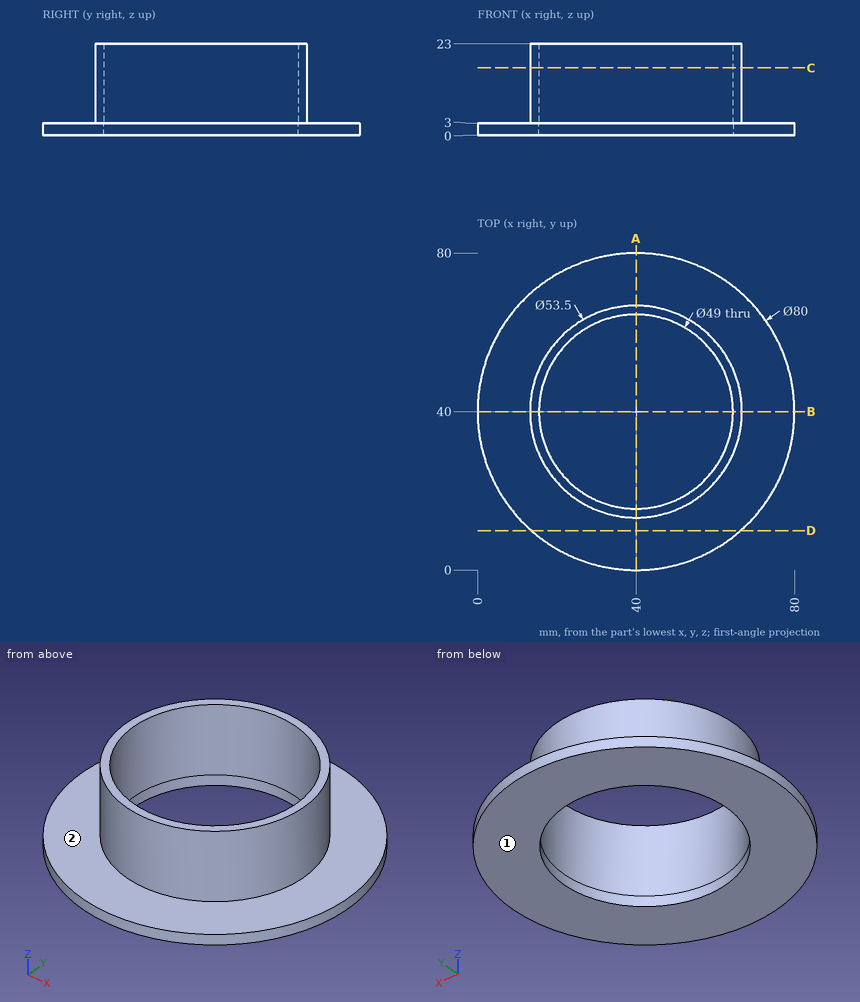
Geometry check sheet. Reference: drawing and pictorial views, mm from the part's lowest x, y, z. A direction names the side the tool comes from. Give positions to 0.01 mm unless a question says otherwise; leave off trailing zeros. Loops run counter-clockwise (first coordinate to the right, second up) from the corner with the lowest first, then second, coordinate; pieces in that order, holes last. Notation, with made-up numbers: (-30, 72.5) - (22, 72.5) arc R5 cw to (22, 79.5) - close; hole circle Ø4 at (12, 8). An arc over 180 degrees is marked (long way). One line per question, with ' | ' between items. Start each with the question number.
1. Cross-section at D-D, the plane y = 10. Enter the section's corners in (x, z).
2. Cross-section at C-C, the plane z = 17. Enter the section's corners in (x, y).
3. Cross-section at A-A, the plane x = 40. Enter the section's corners in (y, z).
4. Set-up check for the marked faces 1 and 2: record each of +Z, -Z, +X, -X, +Y, -Y from which the full face is reachable in a straight line by a thin tool's end or side.
5. Material ranges on line 1 along Y through (x, z) = (40, 8.5); line 2 along Y through (x, z) = (40, 0.85); line 3 along Z through (x, y) = (72, 46.5), recorded low to high. Write a range as [from, to].
6. Gauge pin test, flat ends, axial feed: pin 1 Ø12 at (x, z) = (66.5, 16) entering from -Y; pin 2 Ø8 at (y, z) = (27.5, 12) entering from +X; pin 3 Ø1 at (y, z) = (58, 6) entering from +X; pin 4 Ø1.5 at (y, z) = (68, 6.5) entering from -X. Record the tip position at first contact, or that the pin passes through.
Check result:
1) outline: (13.54, 0) - (66.46, 0) - (66.46, 3) - (13.54, 3) - close
2) outline: circle Ø53.5 at (40, 40); hole circle Ø49 at (40, 40)
3) outline: (0, 0) - (15.5, 0) - (15.5, 23) - (13.25, 23) - (13.25, 3) - (0, 3) - close; (64.5, 0) - (80, 0) - (80, 3) - (66.75, 3) - (66.75, 23) - (64.5, 23) - close
4) face 1: -Z, +X, -X, +Y, -Y | face 2: +Z
5) line 1: y = [13.25, 15.5], [64.5, 66.75] | line 2: y = [0, 15.5], [64.5, 80] | line 3: z = [0, 3]
6) pin 1: stops at y = 22.82 | pin 2: stops at x = 65.36 | pin 3: stops at x = 60.23 | pin 4: passes through
